The model under review builds one solid part; all positions refer to its coordinate system, in mm. A direction names the side the tool comes from. Coordinates: 2 decimals unless noted, no trailing zeros. Write each loop counter-clockwise with the first axis right and the second up, starting at its lowest first coordinate (ties: lowest second). Pieces come first, ordered by that corner, then holes.
1) Add section A-A, the plane z = 24. State the section outline as (x, y) points, then the cut area to 3 significant figures.
2) Machinability: for faces 1 (the cylindrical face through (-38.59, 23.794, 2.419)), 2 (the cylindrical face through (-36.35, 44.37, -28.82)), 3 (the cylindrical face through (-37.395, 44.37, -29.896)), which of the approach directions +Z, -Z, +X, -X, +Y, -Y give a long, thin tool a straight path to every point of the face, cutting with its end or side? Answer none if there is none.
3) Add section B-B, the plane y = 10. State the section outline as (x, z) points.
4) Add section D-D, the plane y = 70. State the section outline as (x, z) points, then the cut area to 3 significant figures.
5) Add section C-C, the plane x = -23.6. Give the number of separate pieces and of enclosed holes in the cut face, then the cut area to 3 significant figures.
6) For line 1 (Y direction, x = -23.6, z = 30.8); line 2 (Z direction, x = 32.5, y = 12); line 3 (X direction, y = 37.5, z = 6), list the stretches that pass through material, from the lowest coordinate up.
7) Mouldability with a two-part tool opening along X and no side actions: class faces 4 (the cylindrical face through (37.496, 44.37, -29.795)), 5 (the cylindrical face through (-26.92, 13.04, 31.01)), 6 (the cylindrical face through (-24.19, 84.46, -30.99)), 7 (the cylindrical face through (-38.59, 74.46, -0.59)) as released by +X, released by -X, zero draft, split by the parting line, or undercut.
8) For P1, Ø8, axis at x = -23.6, y = 10, coming from the +Z side, flat-tipped, find the tip position at first contact; note if it passes through.
from build123d import *

# Parameters (mm, degrees)
BOSS_EXTRUDE1_DEPTH = 90
SKETCH2_R           = 4.5
CUT_EXTRUDE1_DEPTH  = 17
SKETCH3_R           = 4.5
CUT_EXTRUDE2_DEPTH  = 95
CUT_EXTRUDE3_DEPTH  = 29


with BuildPart() as part:
    # Sketch1 → Boss-Extrude1 (new body)
    with BuildSketch(Plane(origin=(0, 0, 0), x_dir=(1, 0, 0), z_dir=(0, 1, 0))):
        with BuildLine():
            Line((-32.85, -31.75), (32.85, -31.75))
            ThreePointArc((32.85, -31.75), (37.446194078, -29.846194078), (39.35, -25.25))
            Line((39.35, -25.25), (39.35, 25.25))
            ThreePointArc((39.35, 25.25), (37.446194078, 29.846194078), (32.85, 31.75))
            Line((32.85, 31.75), (-32.85, 31.75))
            ThreePointArc((-32.85, 31.75), (-37.446194078, 29.846194078), (-39.35, 25.25))
            Line((-39.35, 25.25), (-39.35, -25.25))
            ThreePointArc((-39.35, -25.25), (-37.446194078, -29.846194078), (-32.85, -31.75))
        make_face()
        with BuildLine():
            Line((-32.85, -30.25), (32.85, -30.25))
            ThreePointArc((32.85, -30.25), (36.385533906, -28.785533906), (37.85, -25.25))
            Line((37.85, -25.25), (37.85, 25.25))
            ThreePointArc((37.85, 25.25), (36.385533906, 28.785533906), (32.85, 30.25))
            Line((32.85, 30.25), (-32.85, 30.25))
            ThreePointArc((-32.85, 30.25), (-36.385533906, 28.785533906), (-37.85, 25.25))
            Line((-37.85, 25.25), (-37.85, -25.25))
            ThreePointArc((-37.85, -25.25), (-36.385533906, -28.785533906), (-32.85, -30.25))
        make_face(mode=Mode.SUBTRACT)
    extrude(amount=BOSS_EXTRUDE1_DEPTH)

    # Sketch2 → Cut-Extrude1 (cut)
    with BuildSketch(Plane.ZY.offset(34.75)):
        with Locations((0, 70)):
            Circle(SKETCH2_R)
        with Locations((0, 20)):
            Circle(SKETCH2_R)
    extrude(amount=CUT_EXTRUDE1_DEPTH, mode=Mode.SUBTRACT)

    # Sketch3 → Cut-Extrude2 (cut)
    with BuildSketch(Plane.XY.offset(32.25)):
        with Locations((-23.6, 80)):
            Circle(SKETCH3_R)
        with Locations((-23.6, 10)):
            Circle(SKETCH3_R)
        with Locations((-23.6, 45)):
            Circle(SKETCH3_R)
    extrude(amount=-CUT_EXTRUDE2_DEPTH, mode=Mode.SUBTRACT)

    # Sketch4 → Cut-Extrude3 (cut)
    with BuildSketch(Plane(origin=(34.75, 0, 0), x_dir=(0, 0, -1), z_dir=(1, 0, 0))):
        with BuildLine():
            Line((-17.5, 82), (17.5, 82))
            ThreePointArc((17.5, 82), (19.5, 80), (17.5, 78))
            Line((17.5, 78), (-17.5, 78))
            ThreePointArc((-17.5, 78), (-19.5, 80), (-17.5, 82))
        make_face()
        with BuildLine():
            Line((-17.5, 72), (17.5, 72))
            ThreePointArc((17.5, 72), (19.5, 70), (17.5, 68))
            Line((17.5, 68), (-17.5, 68))
            ThreePointArc((-17.5, 68), (-19.5, 70), (-17.5, 72))
        make_face()
        with BuildLine():
            Line((-17.5, 62), (17.5, 62))
            ThreePointArc((17.5, 62), (19.5, 60), (17.5, 58))
            Line((17.5, 58), (-17.5, 58))
            ThreePointArc((-17.5, 58), (-19.5, 60), (-17.5, 62))
        make_face()
        with BuildLine():
            Line((-17.5, 52), (17.5, 52))
            ThreePointArc((17.5, 52), (19.5, 50), (17.5, 48))
            Line((17.5, 48), (-17.5, 48))
            ThreePointArc((-17.5, 48), (-19.5, 50), (-17.5, 52))
        make_face()
        with BuildLine():
            Line((-17.5, 42), (17.5, 42))
            ThreePointArc((17.5, 42), (19.5, 40), (17.5, 38))
            Line((17.5, 38), (-17.5, 38))
            ThreePointArc((-17.5, 38), (-19.5, 40), (-17.5, 42))
        make_face()
        with BuildLine():
            Line((-17.5, 32), (17.5, 32))
            ThreePointArc((17.5, 32), (19.5, 30), (17.5, 28))
            Line((17.5, 28), (-17.5, 28))
            ThreePointArc((-17.5, 28), (-19.5, 30), (-17.5, 32))
        make_face()
        with BuildLine():
            Line((-17.5, 22), (17.5, 22))
            ThreePointArc((17.5, 22), (19.5, 20), (17.5, 18))
            Line((17.5, 18), (-17.5, 18))
            ThreePointArc((-17.5, 18), (-19.5, 20), (-17.5, 22))
        make_face()
        with BuildLine():
            Line((-17.5, 12), (17.5, 12))
            ThreePointArc((17.5, 12), (19.5, 10), (17.5, 8))
            Line((17.5, 8), (-17.5, 8))
            ThreePointArc((-17.5, 8), (-19.5, 10), (-17.5, 12))
        make_face()
    extrude(amount=CUT_EXTRUDE3_DEPTH, mode=Mode.SUBTRACT)


solid = part.part
Geometry results:
1. outline: (-39.35, 0) - (-37.85, 0) - (-37.85, 90) - (-39.35, 90) - close; (37.85, 0) - (39.35, 0) - (39.35, 90) - (37.85, 90) - close
1. area: 270 mm2
2. face 1: -X
2. face 2: +Y, -Y
2. face 3: -Z, -X, +Y, -Y
3. outline: (-39.35, -25.25) arc R6.5 ccw to (-32.85, -31.75) - (-28.1, -31.75) - (-28.1, -30.25) - (-32.85, -30.25) arc R5 cw to (-37.85, -25.25) - (-37.85, 25.25) arc R5 cw to (-32.85, 30.25) - (-28.1, 30.25) - (-28.1, 31.75) - (-32.85, 31.75) arc R6.5 ccw to (-39.35, 25.25) - close; (-19.1, -31.75) - (32.85, -31.75) arc R6.5 ccw to (39.35, -25.25) - (39.35, -19.5) - (37.85, -19.5) - (37.85, -25.25) arc R5 cw to (32.85, -30.25) - (-19.1, -30.25) - close; (-19.1, 30.25) - (32.85, 30.25) arc R5 cw to (37.85, 25.25) - (37.85, 19.5) - (39.35, 19.5) - (39.35, 25.25) arc R6.5 ccw to (32.85, 31.75) - (-19.1, 31.75) - close
4. outline: (-39.35, -25.25) arc R6.5 ccw to (-32.85, -31.75) - (32.85, -31.75) arc R6.5 ccw to (39.35, -25.25) - (39.35, -19.5) - (37.85, -19.5) - (37.85, -25.25) arc R5 cw to (32.85, -30.25) - (-32.85, -30.25) arc R5 cw to (-37.85, -25.25) - (-37.85, -4.5) - (-39.35, -4.5) - close; (-39.35, 4.5) - (-37.85, 4.5) - (-37.85, 25.25) arc R5 cw to (-32.85, 30.25) - (32.85, 30.25) arc R5 cw to (37.85, 25.25) - (37.85, 19.5) - (39.35, 19.5) - (39.35, 25.25) arc R6.5 ccw to (32.85, 31.75) - (-32.85, 31.75) arc R6.5 ccw to (-39.35, 25.25) - close
4. area: 331 mm2
5. separate pieces: 8
5. enclosed holes: 0
5. area: 189 mm2
6. line 1: y = 0 to 5.5, 14.5 to 40.5, 49.5 to 75.5, 84.5 to 90
6. line 2: z = -31.75 to -30.25, 30.25 to 31.75
6. line 3: x = -39.35 to -37.85, 37.85 to 39.35
7. face 4: released by +X
7. face 5: undercut
7. face 6: undercut
7. face 7: zero draft
8. P1: passes through
